Read the model definition and answer for the solid it produces. Units are mm, in the model's axes. Coordinates: 2 decimals unless noted, no trailing zeros. Loops run counter-clockwise (first coordinate to the right, second up) from the corner with the lowest first, then second, coordinate; pieces in that order, holes last.
Autodesk Inventor part; units mm, degrees
ref_plane "YZ Plane" through (0, 0, 0) normal (1, 0, 0) x (0, 1, 0)
ref_plane "XZ Plane" through (0, 0, 0) normal (0, 1, 0) x (-1, 0, 0)
ref_plane "XY Plane" through (0, 0, 0) normal (0, 0, 1) x (1, 0, 0)
sketch "Sketch4" plane through (0, 0, 0) normal (0, 0, 1) x (1, 0, 0)
  line L0 (0, 0) -> (-40, 0)
  line L1 (-40, 0) -> (-40, 40)
  line L2 (-40, 40) -> (0, 40)
  line L3 (0, 40) -> (0, 0)
  dimension "d37" = 40
  dimension "d38" = 40
extrude "Extrusion2" add sketch "Sketch4" along normal blind 14
hole "Hole3" at (-30, 35, 14) direction (0, 0, -1) diameter 4.917 depth 17.1 tip angle 118
hole "Hole4" at (-10, 35, 14) direction (0, 0, -1) diameter 4.917 depth 17.1 tip angle 118
hole "Hole5" at (-10, 5, 14) direction (0, 0, -1) diameter 4.978 depth 19.05 tip angle 118
hole "Hole6" at (-30, 5, 14) direction (0, 0, -1) diameter 4.917 depth 17.1 tip angle 118
hole "Hole7" at (0, 20, -1) direction (-1, 0, 0) diameter 19 end through all
fillet "Fillet1" radius 5 4 edges at (-40, 40, 7) (0, 40, 7) (0, 0, 7) (-40, 0, 7)
properties part number "GARFO" material "Aluminium AW-7020"
Item 1: A cutting plane is placed at B-B on x = -10. Determine the outline of the cut face in (y, z).
Numbers:
outline: (0, 0) - (2.51, 0) - (2.51, 14) - (0, 14) - close; (7.49, 0) - (10.55, 0) arc R9.5 cw to (29.45, 0) - (32.54, 0) - (32.54, 14) - (7.49, 14) - close; (37.46, 0) - (40, 0) - (40, 14) - (37.46, 14) - close
Item 2: A cutting plane is placed at C-C on z = 11. Determine the outline of the cut face in (x, y), then the cut area to 3 significant figures.
Numbers:
outline: (-40, 5) arc R5 ccw to (-35, 0) - (-5, 0) arc R5 ccw to (0, 5) - (0, 35) arc R5 ccw to (-5, 40) - (-35, 40) arc R5 ccw to (-40, 35) - close; hole circle Ø4.92 at (-30, 5); hole circle Ø4.92 at (-30, 35); hole circle Ø4.98 at (-10, 5); hole circle Ø4.92 at (-10, 35)
area: 1,500 mm2
Item 3: Given pin 1 (4 mm diameter, centred on x = -30, y = 5, fed in from -Z); pin 2 (6 mm diameter, centred on x = -17, y = 22.5, fed in from -Z); pin 3 (1 mm diameter, centred on x = -12.5, y = 28, fed in from -Z); pin 4 (3 mm diameter, centred on x = -30, y = 23, fed in from -Z), each flat-ended and moving along its own axis, determine where each tip first touches the part or whether it passes through.
Numbers:
pin 1: passes through
pin 2: stops at z = 6.75
pin 3: stops at z = 3.24
pin 4: stops at z = 7.37
Item 4: A cutting plane is placed at A-A on z = 5.5. Determine the outline of the cut face in (x, y), then the cut area to 3 significant figures.
Numbers:
outline: (-40, 5) arc R5 ccw to (-35, 0) - (-5, 0) arc R5 ccw to (0, 5) - (0, 13.07) - (-40, 13.07) - close; (-40, 26.93) - (0, 26.93) - (0, 35) arc R5 ccw to (-5, 40) - (-35, 40) arc R5 ccw to (-40, 35) - close; hole circle Ø4.92 at (-30, 5); hole circle Ø4.92 at (-30, 35); hole circle Ø4.98 at (-10, 5); hole circle Ø4.92 at (-10, 35)
area: 948 mm2
Item 5: Determine the mould class of faces 1 (the face through (-27.6, 5.53, 6.9)), 2 (the face through (-1, 38, 7)), 3 (the face through (-20, 40, 7)) for opening direction X: released by +X, released by -X, zero draft, split by the parting line, or undercut.
Numbers:
face 1: undercut
face 2: released by +X
face 3: zero draft
Item 6: A cutting plane is placed at D-D on x = -27. Determine the outline of the cut face in (y, z), then the cut area to 3 significant figures.
Numbers:
outline: (0, 0) - (10.55, 0) arc R9.5 cw to (29.45, 0) - (40, 0) - (40, 14) - (0, 14) - close
area: 437 mm2
Item 7: Find the intervals of material crossed by line 1 along X through (y, z) = (5, 6.5); line 2 along Y through (x, z) = (-11, 2); line 3 along Y through (x, z) = (-30, 4.25), in increasing order.
Numbers:
line 1: x = -40 to -32.46, -27.54 to -12.49, -7.51 to 0
line 2: y = 0 to 2.72, 7.28 to 10.99, 29.01 to 32.75, 37.25 to 40
line 3: y = 0 to 2.54, 7.46 to 12.08, 27.92 to 32.54, 37.46 to 40
